```python
from build123d import *

# Parameters (mm, degrees)
SKETCH5_R             = 1.27
BOSS_EXTRUDE2_DEPTH   = 2.54
BOSS_EXTRUDE2_2_DEPTH = 2.54
BOSS_EXTRUDE1_DEPTH   = 5.08
SKETCH6_R             = 3.175
BOSS_EXTRUDE3_DEPTH   = 7.62
SKETCH11_R            = 19.05
BOSS_EXTRUDE4_DEPTH   = 5.08
SKETCH13_R            = 19.05
BOSS_EXTRUDE5_DEPTH   = 5.08


with BuildPart() as part:
    # Sketch5 → Boss-Extrude2 (new body)
    with BuildSketch(Plane(origin=(0, 0, 0), x_dir=(1, 0, 0), z_dir=(0, 1, 0))):
        Polygon((-22.86, 10.16), (-22.86, -10.16), (-17.78, -12.417777778), (-17.78, 12.417777778), align=None)
        with Locations(Location((-20.32, 0, 0), (0, 0, 270))):
            Circle(SKETCH5_R, mode=Mode.SUBTRACT)
    extrude(amount=BOSS_EXTRUDE2_DEPTH)



with BuildPart() as body_2:
    # Sketch5 → Boss-Extrude2 2 (new body)
    with BuildSketch(Plane(origin=(0, 0, 0), x_dir=(1, 0, 0), z_dir=(0, 1, 0))):
        Polygon((22.86, 10.16), (17.78, 12.417777778), (17.78, -12.417777778), (22.86, -10.16), align=None)
        with Locations(Location((20.32, 0, 0), (0, 0, 90))):
            Circle(SKETCH5_R, mode=Mode.SUBTRACT)
    extrude(amount=BOSS_EXTRUDE2_2_DEPTH)


with BuildPart() as part_1:
    add(part.part)

    add(body_2.part)  # Boss-Extrude1 merges body 2
    # Sketch2 → Boss-Extrude1 (add)
    with BuildSketch(Plane(origin=(0, 0, 0), x_dir=(1, 0, 0), z_dir=(0, 1, 0))):
        with BuildLine():
            Line((-53.071845065, -4.54369013), (-2.271845065, -29.94369013))
            ThreePointArc((-2.271845065, -29.94369013), (0, -30.48), (2.271845065, -29.94369013))
            Line((2.271845065, -29.94369013), (53.071845065, -4.54369013))
            ThreePointArc((53.071845065, -4.54369013), (55.88, 0), (53.071845065, 4.54369013))
            Line((53.071845065, 4.54369013), (2.271845065, 29.94369013))
            ThreePointArc((2.271845065, 29.94369013), (0, 30.48), (-2.271845065, 29.94369013))
            Line((-2.271845065, 29.94369013), (-53.071845065, 4.54369013))
            ThreePointArc((-53.071845065, 4.54369013), (-55.88, 0), (-53.071845065, -4.54369013))
        make_face()
        Polygon((-45.72, 0), (0, 20.32), (45.72, 0), (0, -20.32), align=None, mode=Mode.SUBTRACT)
    extrude(amount=BOSS_EXTRUDE1_DEPTH)

    # Sketch6 → Boss-Extrude3 (add)
    with BuildSketch(Plane(origin=(0, 5.08, 0), x_dir=(1, 0, 0), z_dir=(0, 1, 0))):
        with Locations(Location((-50.8, 0, 0), (0, 0, 90))):
            Circle(SKETCH6_R)
        with Locations(Location((50.8, 0, 0), (0, 0, 90))):
            Circle(SKETCH6_R)
    extrude(amount=BOSS_EXTRUDE3_DEPTH)

    # Sketch11 → Boss-Extrude4 (add)
    with BuildSketch(Plane(origin=(0, 12.7, 0), x_dir=(1, 0, 0), z_dir=(0, 1, 0))):
        with Locations(Location((-50.8, 0, 0), (0, 0, 270))):
            Circle(SKETCH11_R)
    extrude(amount=BOSS_EXTRUDE4_DEPTH)

    # Sketch13 → Boss-Extrude5 (add)
    with BuildSketch(Plane(origin=(0, 12.7, 0), x_dir=(1, 0, 0), z_dir=(0, 1, 0))):
        with Locations(Location((50.8, 0, 0), (0, 0, 270))):
            Circle(SKETCH13_R)
    extrude(amount=BOSS_EXTRUDE5_DEPTH)


solid = part_1.part
```
For this review, take the finished solid that the model builds, in its own axes (mm). A direction names the side the tool comes from. Give positions to 0.01 mm unless a question says otherwise; leave off trailing zeros. Loops run counter-clockwise (first coordinate to the right, second up) from the corner with the lowest first, then second, coordinate; pieces in that order, holes last. Notation, with made-up numbers: M 80.25,7.25 L 132.25,7.25 A18 ccw 132.25,19.25 Z; hole C 71,86 d3. An arc over 180 degrees is marked long. One line per item, written item: value. Start each with the question number.
Q1. Machinability: for faces 4 (the face through (28.027, 2.504, -17.066)), 5 (the face through (-18.7, 2.54, -0.2)), 6 (the face through (-55.88, 2.5, -0.08)), 7 (the face through (-53.95, 8.84, 0.41)), 8 (the face through (17.78, 1, 0)), which of the approach directions +Z, -Z, +X, -X, +Y, -Y give a long, thin tool a straight path to every point of the face, cutting with its end or side? Answer none if there is none.
Q2. Draft analysis for pull direction Y (two halves, no side actions). For faces 1 (the face through (51, 17.78, 0)), 2 (the face through (47.65, 8.84, 0.41)), 3 (the face through (22.86, 1, 0)), state which applies: released by +Y, released by -Y, zero draft, split by the parting line, or undercut.
Q3. Add section B-B (y = 14). Give the boundary of the cut face in (x, z), and give its area (3 significant figures).
Q4. Add section C-C (z = 8.5). Give the boundary of the cut face in (x, y) (3 decimals), and give its area (3 significant figures).
Q5. Add section A-A (x = -20.32). Give the boundary of the cut face in (y, z).
Q6. Clearance check with flat-ended pins moving along their axes: pin 1 Ø1.5 at (x, z) = (-20.32, 0) entering from -Y; pin 2 Ø1.5 at (x, z) = (50, -2) entering from -Y; pin 3 Ø5 at (x, y) = (-45.5, 13) entering from +Z; pin 4 Ø1 at (x, y) = (22.5, 5.5) entering from +Z. State where each tip first meets the part, or that it passes through.
Q7. Add section D-D (x = 4). Give the boundary of the cut face in (y, z).
Q8. For L1, parallel to Y at x = 36, z = 6; L2, parallel to Y at x = -36.5, z = 0; L3, parallel to X at y = 16.5, z = 7.5, list the stretches that pass through material, from the lowest coordinate up.
Reply:
1. face 4: -Z, +X, -Y
1. face 5: +Y
1. face 6: -X, -Y
1. face 7: none
1. face 8: +Y, -Y
2. face 1: released by +Y
2. face 2: undercut
2. face 3: zero draft
3. outline: C -50.8,0 d38.1; C 50.8,0 d38.1
3. area: 2,280 mm²
4. outline: M -67.849,12.7 L -33.751,12.7 L -33.751,17.78 L -67.849,17.78 Z; M -45.159,0 L -26.595,0 L -26.595,5.08 L -45.159,5.08 Z; M -22.86,0 L -17.78,0 L -17.78,2.54 L -22.86,2.54 Z; M 17.78,0 L 22.86,0 L 22.86,2.54 L 17.78,2.54 Z; M 26.595,0 L 45.159,0 L 45.159,5.08 L 26.595,5.08 Z; M 33.751,12.7 L 67.849,12.7 L 67.849,17.78 L 33.751,17.78 Z
4. area: 561 mm²
5. outline: M 0,-20.92 L 5.08,-20.92 L 5.08,-11.29 L 2.54,-11.29 L 2.54,-1.27 L 0,-1.27 Z; M 0,1.27 L 2.54,1.27 L 2.54,11.29 L 5.08,11.29 L 5.08,20.92 L 0,20.92 Z
6. pin 1: through
6. pin 2: y = 0
6. pin 3: z = 18.84
6. pin 4: z = 19.97
7. outline: M 0,-29.08 L 5.08,-29.08 L 5.08,-18.54 L 0,-18.54 Z; M 0,18.54 L 5.08,18.54 L 5.08,29.08 L 0,29.08 Z
8. L1: 0 to 5.08, 12.7 to 17.78
8. L2: 12.7 to 17.78
8. L3: -68.31 to -33.29, 33.29 to 68.31
